Could you check a few things on this drawing? It's one solid part, dimensions in mm from its lowest x, y, z. A direction names the side the tool comes from. Give positions to 0.01 mm unless a question says otherwise; leave off trailing zeros. Order: outer loops, then holes, each group sorted by start corner. A loop starts at its lowest first (then second) coordinate and runs counter-clockwise, first axis right, second up. Notation, with made-up numbers: (43, 63) - (94, 63) arc R28 cw to (94, 101) - close; hole circle Ø9 at (56, 52). An arc over 180 degrees is marked (long way). Put each result on its own line as item: value.
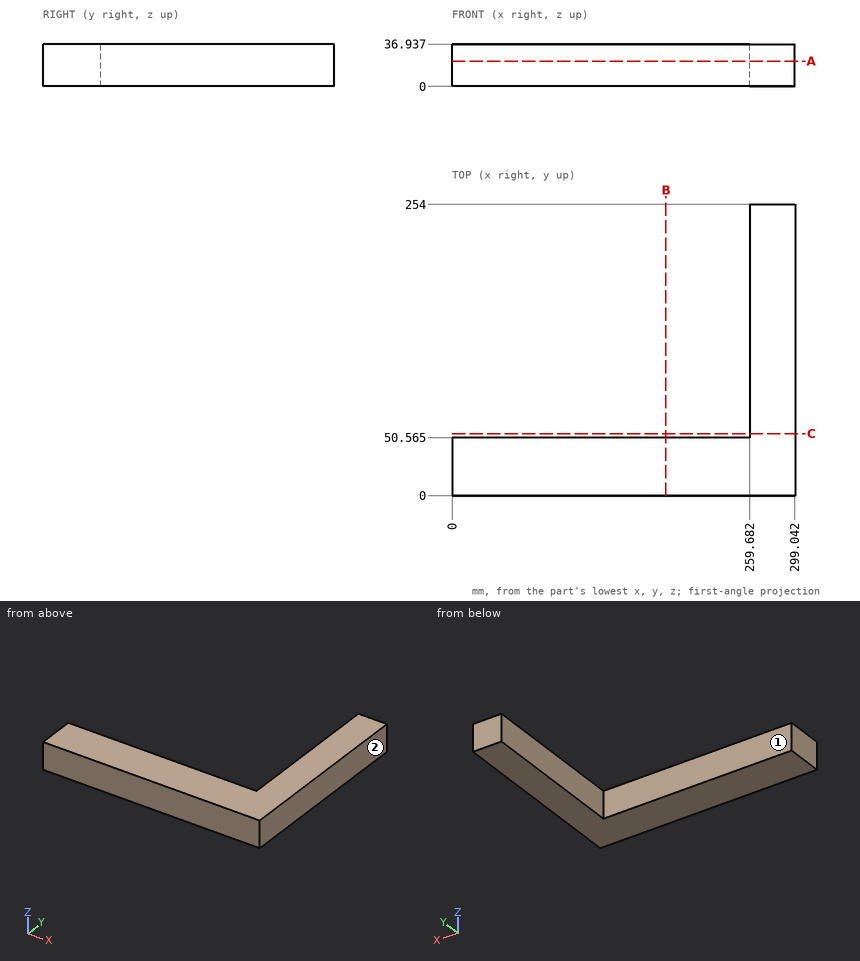
1) Suppose I cut it at A-A, the plane z = 22. List the corners of the cut face in (x, y) for me (1 decimal), and give its area (3 significant figures).
Filled in:
outline: (0, 0) - (299, 0) - (299, 254) - (259.7, 254) - (259.7, 50.6) - (0, 50.6) - close
area: 23,100 mm^2
2) Suppose I cut it at B-B, the plane x = 186.5. List the corners of the cut face in (y, z) for me (1 decimal), and give its area (3 significant figures).
Filled in:
outline: (0, 0) - (50.6, 0) - (50.6, 36.9) - (0, 36.9) - close
area: 1,870 mm^2
3) Suppose I cut it at C-C, the plane y = 54. List the corners of the cut face in (x, z) for me.
Filled in:
outline: (259.68, 0) - (299.04, 0) - (299.04, 36.94) - (259.68, 36.94) - close
4) Which directions (+Z, -Z, +X, -X, +Y, -Y) give clear straight access to the entire face, cutting with the end or side of a thin tool? Please do the marked faces 1 and 2.
Filled in:
face 1: +Z, -Z, -X, +Y
face 2: +Z, -Z, +X, +Y, -Y
5) If I drill on line 1 (Y direction, x = 154, z = 25) (1 decimal); line 2 (X direction, y = 216.5, z = 23.5), over which ranges is the centre line in solid material (lowest first)? Write a range as [from, to].
Filled in:
line 1: y = [0, 50.6]
line 2: x = [259.68, 299.04]
6) I'm going to push flat-ended pins straight in: pin 1 (12 mm diameter, centred on y = 227.5, z = 11, fed in from -X); pin 2 (3 mm diameter, centred on x = 202.5, z = 26.5, fed in from +Y) (1 decimal). Where does each tip first touch, or does it pass through?
Filled in:
pin 1: stops at x = 259.68
pin 2: stops at y = 50.6
